Source: CAD feature listing. Evaluate the final solid. Frame: model axes, mm. A direction names the side the tool comes from. Coordinates: 2 decimals unless noted, no trailing zeros. Loops run counter-clockwise (first coordinate to the right, second up) from the corner with the lowest first, then second, coordinate; pieces in that order, holes last. Notation, with made-up numbers: (72, 84.5) - (111, 84.5) arc R19 ccw to (111, 100.5) - close; hole circle Ø5 at (-35.5, 27). An arc over 180 degrees is marked (long way). Write item = value, one per line. Start each with the question number.
from build123d import *

# Parameters (mm, degrees)
BOSS_EXTRU_2_DEPTH      = 11.5
ESQUISSE2_W             = 64
ESQUISSE2_H             = 3.5
BOSS_EXTRU_3_DEPTH      = 10
CONG_1_R                = 10
ESQUISSE3_R             = 1.1
ENL_V_MAT_EXTRU_1_DEPTH = 4.5
ENL_V_MAT_EXTRU_2_DEPTH = 1.4


with BuildPart() as part:
    # Esquisse1 → Boss.-Extru.2 (new body)
    with BuildSketch(Plane.XY):
        with BuildLine():
            Line((-32, 10.25), (-24.5, 10.25))
            ThreePointArc((-24.5, 10.25), (-24.212828793, 9.792463035), (-24.5, 9.334926071))
            ThreePointArc((-24.5, 9.334926071), (-20.5, -8.15), (-16.5, 9.334926071))
            ThreePointArc((-16.5, 9.334926071), (-16.787171207, 9.792463035), (-16.5, 10.25))
            Line((-16.5, 10.25), (-4, 10.25))
            ThreePointArc((-4, 10.25), (-3.712828793, 9.792463035), (-4, 9.334926071))
            ThreePointArc((-4, 9.334926071), (0, -8.15), (4, 9.334926071))
            ThreePointArc((4, 9.334926071), (3.712828793, 9.792463035), (4, 10.25))
            Line((4, 10.25), (16.5, 10.25))
            ThreePointArc((16.5, 10.25), (16.787171207, 9.792463035), (16.5, 9.334926071))
            ThreePointArc((16.5, 9.334926071), (20.5, -8.15), (24.5, 9.334926071))
            ThreePointArc((24.5, 9.334926071), (24.212828793, 9.792463035), (24.5, 10.25))
            Line((24.5, 10.25), (32, 10.25))
            Line((32, 10.25), (32, -0.25))
            ThreePointArc((32, -0.25), (29.071067812, -7.321067812), (22, -10.25))
            Line((22, -10.25), (-22, -10.25))
            ThreePointArc((-22, -10.25), (-29.071067812, -7.321067812), (-32, -0.25))
            Line((-32, -0.25), (-32, 10.25))
        make_face()
    extrude(amount=BOSS_EXTRU_2_DEPTH)

    # Esquisse2 → Boss.-Extru.3 (add)
    with BuildSketch(Plane.XY.offset(11.5)):
        with Locations((0, 8.5)):
            Rectangle(ESQUISSE2_W, ESQUISSE2_H)
    extrude(amount=BOSS_EXTRU_3_DEPTH)

    # Congé1
    cong_1_edges = [part.edges().sort_by_distance(p)[0] for p in [
        (32, 8.5, 21.5),
        (-32, 8.5, 21.5),
    ]]
    fillet(cong_1_edges, radius=CONG_1_R)

    # Esquisse3 → Enlèv. mat.-Extru.1 (cut, through all)
    with BuildSketch(Plane.XZ.offset(-6.75)):
        with Locations((-22, 16.5)):
            Circle(ESQUISSE3_R)
        with Locations((22, 16.5)):
            Circle(ESQUISSE3_R)
    extrude(amount=-ENL_V_MAT_EXTRU_1_DEPTH, mode=Mode.SUBTRACT)

    # Esquisse4 → Enlèv. mat.-Extru.2 (cut)
    with BuildSketch(Plane.XZ.offset(-6.75)):
        Polygon((-20.845299462, 14.5), (-19.690598923, 16.5), (-20.845299462, 18.5), (-23.154700538, 18.5), (-24.309401077, 16.5), (-23.154700538, 14.5), align=None)
        Polygon((24.309401077, 16.5), (23.154700538, 18.5), (20.845299462, 18.5), (19.690598923, 16.5), (20.845299462, 14.5), (23.154700538, 14.5), align=None)
    extrude(amount=-ENL_V_MAT_EXTRU_2_DEPTH, mode=Mode.SUBTRACT)


solid = part.part
Item 1: Draft query along Y for faces 5 (the flat face through (-21, 8.15, 17.4)), 6 (the cylindrical face through (29.15, 8.52, 18.49)), 7 (the flat face through (20, 8, 11.5)). Return one class per face: released by +Y, released by -Y, zero draft, split by the parting line, or undercut.
Item 2: First-contact query: pin 1 (3 mm diameter, centred on x = 6, y = -1.5, fed in from +Z); pin 2 (4 mm diameter, centred on x = 0.5, y = 8.5, fed in from -Z); pin 3 (3.5 mm diameter, centred on x = 22, z = 16.5, fed in from -Y). Flat tips, straight axial feed; report the tip coordinate or a pass-through.
Item 3: Cut plane B-B (y = 1.05). Return the cut outline in (x, z), then the cut area to 3 significant figures.
Item 4: Cut plane D-D (y = 6). Return the cut outline in (x, z).
Item 5: Reachability of faces 1 (the flat face through (-2, -9, 11.5)), 2 (the flat face through (-23.74, 7.44, 15.51)), 3 (the cylindrical face through (-22.87, 9.19, 15.83)), 4 (the cylindrical face through (-20.847, -8.143, 5.67)) from +Z, -Z, +X, -X, +Y, -Y: full face, straight path, thin tool, end or side. Return the list, or none.
Item 6: Cut plane A-A (x = 0). Return the cut outline in (y, z), then the cut area to 4 significant figures.
Item 7: Cut plane C-C (z = 9). Return the cut outline in (x, y), then the cut area to 3 significant figures.
Item 8: Material intervals for L1, parallel to X at y = 1.05, z = 3.5; L2, parallel to Z at x = 22, y = 9.5; L3, parallel to X at y = -1.5, z = 7.25, sorted ascending. Write a range as [from, to].
Responses:
q1.face_5 = released by -Y
q1.face_6 = zero draft
q1.face_7 = undercut
q2.pin_1 = through
q2.pin_2 = 11.5
q2.pin_3 = 8.15
q3.outline = (-32, 0) - (-29.7, 0) - (-29.7, 11.5) - (-32, 11.5) - close; (-11.3, 0) - (-9.2, 0) - (-9.2, 11.5) - (-11.3, 11.5) - close; (9.2, 0) - (11.3, 0) - (11.3, 11.5) - (9.2, 11.5) - close; (29.7, 0) - (32, 0) - (32, 11.5) - (29.7, 11.5) - close
q3.area = 101 mm2
q4.outline = (-32, 0) - (-28.25, 0) - (-28.25, 11.5) - (-32, 11.5) - close; (-12.75, 0) - (-7.75, 0) - (-7.75, 11.5) - (-12.75, 11.5) - close; (7.75, 0) - (12.75, 0) - (12.75, 11.5) - (7.75, 11.5) - close; (28.25, 0) - (32, 0) - (32, 11.5) - (28.25, 11.5) - close
q5.face_1 = +Z, +X, -X, -Y
q5.face_2 = -Y
q5.face_3 = +Y, -Y
q5.face_4 = -Z
q6.outline = (-10.25, 0) - (-8.15, 0) - (-8.15, 11.5) - (-10.25, 11.5) - close; (6.75, 11.5) - (10.25, 11.5) - (10.25, 21.5) - (6.75, 21.5) - close
q6.area = 59.15 mm2
q7.outline = (-32, -0.25) arc R10 ccw to (-22, -10.25) - (22, -10.25) arc R10 ccw to (32, -0.25) - (32, 10.25) - (24.5, 10.25) arc R0.51 ccw to (24.5, 9.33) arc R9.2 cw (long way) to (16.5, 9.33) arc R0.51 ccw to (16.5, 10.25) - (4, 10.25) arc R0.51 ccw to (4, 9.33) arc R9.2 cw (long way) to (-4, 9.33) arc R0.51 ccw to (-4, 10.25) - (-16.5, 10.25) arc R0.51 ccw to (-16.5, 9.33) arc R9.2 cw (long way) to (-24.5, 9.33) arc R0.51 ccw to (-24.5, 10.25) - (-32, 10.25) - close
q7.area = 465 mm2
q8.L1 = [-32, -29.7], [-11.3, -9.2], [9.2, 11.3], [29.7, 32]
q8.L2 = [11.5, 15.4], [17.6, 21.5]
q8.L3 = [-31.92, -29.34], [-11.66, -8.84], [8.84, 11.66], [29.34, 31.92]
